Work out the finished part from the listing and answer in its coordinate system (mm). A direction names the side the tool comes from. Round coordinates to 2 decimals unless told otherwise and drop trailing zeros. Loops run counter-clockwise (first coordinate to the right, second up) from the corner with the lowest first, then second, coordinate; pieces in that order, holes last.
Autodesk Inventor part; units mm, degrees
ref_plane "YZ Plane" through (0, 0, 0) normal (1, 0, 0) x (0, 1, 0)
ref_plane "XZ Plane" through (0, 0, 0) normal (0, 1, 0) x (-1, 0, 0)
ref_plane "XY Plane" through (0, 0, 0) normal (0, 0, 1) x (1, 0, 0)
sketch "Sketch1" plane through (0, 0, 0) normal (0, 1, 0) x (-1, 0, 0)
  line L0 (100, 155) -> (-100, 155)
  line L1 (-100, 155) -> (-100, -155)
  line L2 (-100, -155) -> (100, -155)
  line L3 (100, -155) -> (100, 155)
  point P0 (0, 0)
  point P1 (100, 0)
  point P2 (0, -155)
  dimension "d0" = 200
  dimension "d1" = 310
extrude "Extrusion1" add sketch "Sketch1" along normal blind 3.5
sketch "Sketch3" plane through (0, 3.5, 0) normal (0, 1, 0) x (1, 0, 0)
  line L0 (-80, 135) -> (-65, 135)
  line L1 (-65, 135) -> (-65, 120)
  line L2 (-65, 120) -> (-80, 120)
  line L3 (-80, 120) -> (-80, 135)
  line L4 (-31, 135) -> (-16, 135)
  line L5 (-16, 135) -> (-16, 120)
  line L6 (-16, 120) -> (-31, 120)
  line L7 (-31, 120) -> (-31, 135)
  line L8 (-80, 35.5) -> (-65, 35.5)
  line L9 (-65, 35.5) -> (-65, 20.5)
  line L10 (-65, 20.5) -> (-80, 20.5)
  line L11 (-80, 20.5) -> (-80, 35.5)
  line L12 (-31, 35.5) -> (-16, 35.5)
  line L13 (-16, 35.5) -> (-16, 20.5)
  line L14 (-16, 20.5) -> (-31, 20.5)
  line L15 (-31, 20.5) -> (-31, 35.5)
  line L16 (-80, -64) -> (-65, -64)
  line L17 (-65, -64) -> (-65, -79)
  line L18 (-65, -79) -> (-80, -79)
  line L19 (-80, -79) -> (-80, -64)
  line L20 (-31, -64) -> (-16, -64)
  line L21 (-16, -64) -> (-16, -79)
  line L22 (-16, -79) -> (-31, -79)
  line L23 (-31, -79) -> (-31, -64)
  line L24 (-100, 155) -> (-100, -155)
  line L25 (100, 155) -> (-100, 155)
  point P0 (0, 0)
  dimension "d4" = 15
  dimension "d5" = 15
  dimension "d8" = 49
  dimension "d11" = 99.5
  dimension "d14" = 20
  dimension "d15" = 20
extrude "Extrusion2" cut sketch "Sketch3" against normal blind 0.5
sketch "Sketch4" plane through (0, 3, 0) normal (0, 1, 0) x (1, 0, 0)
  line L0 (-65, 135) -> (-65, 120)
  line L1 (-65, 120) -> (-80, 120)
  line L2 (-65, 35.5) -> (-65, 20.5)
  line L3 (-31, 20.5) -> (-31, 35.5)
  line L4 (-80, -64) -> (-65, -64)
  line L5 (-31, -79) -> (-31, -64)
  point P0 (0, 0)
  point P1 (-69, 28)
  point P2 (-27, 28)
  point P3 (-69, -68)
  point P4 (-27, -68)
  point P5 (-69, 124)
  point P6 (-27, 124)
  point P7 (-65, 28)
  point P8 (-31, 28)
  dimension "d18" = 4
  dimension "d19" = 4
  dimension "d20" = 4
  dimension "d21" = 4
hole "Hole1" at (-69, 3, -28) at (-27, 3, -28) at (-69, 3, 68) at (-27, 3, 68) at (-69, 3, -124) at (-27, 3, -124) direction (0, -1, 0) diameter 3.5 end through all
properties part number "BaseCase"
1. Which of the six approach directions +Z, -Z, +X, -X, +Y, -Y give full straight-line access (tool end or side, diameter ignored) to faces 1 (the face through (1, 0, 2)), 2 (the face through (-73, 3, -28))?
Answer key:
face 1: +Z, -Z, +X, -X, -Y
face 2: +Y
2. Find section A-A (x = -22). Write down the section's boundary in (y, z).
Answer key:
outline: (0, -155) - (3.5, -155) - (3.5, -135) - (3, -135) - (3, -120) - (3.5, -120) - (3.5, -35.5) - (3, -35.5) - (3, -20.5) - (3.5, -20.5) - (3.5, 64) - (3, 64) - (3, 79) - (3.5, 79) - (3.5, 155) - (0, 155) - close
3. Given pin 1 (7.5 mm diameter, centred on x = -71, z = 73.5, fed in from +Y), flat-ended and moving along its own axis, determine where the tip first touches the part or whether it passes through.
Answer key:
pin 1: stops at y = 3
4. Consider probe 1 along Z at (x, y) = (-27, 1.65); probe 2 along X at (y, z) = (1.55, -28). Determine where each line is inside the solid, lowest interval first.
Answer key:
probe 1: z = -155 to -125.75, -122.25 to -29.75, -26.25 to 66.25, 69.75 to 155
probe 2: x = -100 to -70.75, -67.25 to -28.75, -25.25 to 100
